Verification items for the finished model (mm, model axes). Give positions to 0.01 mm unless a question says otherwise; leave off trailing zeros. Loops run counter-clockwise (first coordinate to the right, second up) from the corner with the lowest first, then second, coordinate; pieces in that order, holes last. Notation, with made-up numbers: (72, 60.25) - (119, 60.25) arc R12 ccw to (119, 83.25) - close; hole circle Ø2 at (52.5, 35.5). An arc over 180 degrees is marked (long way). One line per question, with ' | ' between items. Start each with the question number.
1. Thickness scan on line 1 along Y through (x, z) = (0.55, -7) (3 decimals); line 2 along Z through (x, y) = (-0.5, -53.5); line 3 along Y through (x, z) = (0.6, -20) (3 decimals). Record the ranges inside material, lowest first. Write a range as from..to.
2. Depth check by flat-ended pin: pin 1 Ø2.5 at (y, z) = (-14.795, -13) entering from -X. Enter the tip coordinate at first touch or a pass-through.
3. Section check A-A, the plane z = -13. Enter the section's corners in (x, y) (3 decimals).
4. Section check D-D, the plane x = 0.05. Enter the section's corners in (y, z) (3 decimals).
5. Section check B-B, the plane z = -4. Enter the section's corners in (x, y) (3 decimals).
6. Section check C-C, the plane y = -54. Enter the section's corners in (x, z), then the cut area to 3 significant figures.
from build123d import *

# Parameters (mm, degrees)
EXTRUDE_1_DEPTH     = 2
FILLET_1_R          = 2
FILLET_2_R          = 2
FILLET_3_R          = 2
FILLET_4_R          = 2
SKETCH_2_W          = 12
SKETCH_2_H          = 89.95
EXTRUDE_2_DEPTH     = 2
CUT_EXTRUDE_1_DEPTH = 10
SKETCH_6_R          = 1.6
CUT_EXTRUDE_2_DEPTH = 10
SKETCH_7_W          = 10
SKETCH_7_H          = 89.95
EXTRUDE_3_DEPTH     = 2


with BuildPart() as part:
    # 草图1 → 凸台-拉伸1 (new body)
    with BuildSketch(Plane(origin=(-0.79375, 0, 0), x_dir=(0, -1, 0), z_dir=(-1, 0, 0))):
        with BuildLine():
            Line((38.795, 5), (12.795, 5))
            ThreePointArc((12.795, 5), (11.380786438, 4.414213562), (10.795, 3))
            Line((10.795, 3), (10.795, -13))
            ThreePointArc((10.795, -13), (11.380786438, -14.414213562), (12.795, -15))
            Line((12.795, -15), (47.795, -15))
            Line((47.795, -15), (50.77, -0.039144756))
            Line((50.77, -0.039144756), (55.77, -0.039144756))
            Line((55.77, -0.039144756), (60.77, -0.039144756))
            Line((60.77, -0.039144756), (63.745, -15))
            Line((63.745, -15), (98.745, -15))
            ThreePointArc((98.745, -15), (100.159213562, -14.414213562), (100.745, -13))
            Line((100.745, -13), (100.745, 3))
            ThreePointArc((100.745, 3), (100.159213562, 4.414213562), (98.745, 5))
            Line((98.745, 5), (72.745, 5))
            Line((72.745, 5), (38.795, 5))
        make_face()
    extrude(amount=-EXTRUDE_1_DEPTH)

    # 圆角1
    fillet_1_edges = [part.edges().sort_by_distance(p)[0] for p in [
        (0.20625, -47.795, -15),
    ]]
    fillet(fillet_1_edges, radius=FILLET_1_R)

    # 圆角2
    fillet_2_edges = [part.edges().sort_by_distance(p)[0] for p in [
        (0.20625, -50.77, -0.039144756),
    ]]
    fillet(fillet_2_edges, radius=FILLET_2_R)

    # 圆角3
    fillet_3_edges = [part.edges().sort_by_distance(p)[0] for p in [
        (0.20625, -60.77, -0.039144756),
    ]]
    fillet(fillet_3_edges, radius=FILLET_3_R)

    # 圆角4
    fillet_4_edges = [part.edges().sort_by_distance(p)[0] for p in [
        (0.20625, -63.745, -15),
    ]]
    fillet(fillet_4_edges, radius=FILLET_4_R)

    # 草图2 → 凸台-拉伸2 (add)
    with BuildSketch(Plane(origin=(1.20625, 0, 0), x_dir=(0, 0, -1), z_dir=(1, 0, 0))):
        with Locations((-9, -55.77)):
            Rectangle(SKETCH_2_W, SKETCH_2_H)
        Polygon((13.39006724, -48.115138781), (25, -45.806477318), (25, -10.795), (13, -10.795), align=None)
        Polygon((13.39006724, -63.424861219), (25, -65.733522682), (25, -100.745), (13, -100.745), align=None)
    extrude(amount=-EXTRUDE_2_DEPTH)

    # 草图5 → 切除-拉伸1 (cut)
    with BuildSketch(Plane(origin=(1.20625, 0, 0), x_dir=(0, 0, -1), z_dir=(1, 0, 0))):
        Polygon((1.649077515, -50.449861219), (25, -45.806477318), (25, -39.241825321), align=None)
        Polygon((1.649077515, -61.090138781), (25, -72.298174679), (25, -65.733522682), align=None)
    extrude(amount=-CUT_EXTRUDE_1_DEPTH, mode=Mode.SUBTRACT)

    # 草图6 → 切除-拉伸2 (cut)
    with BuildSketch(Plane(origin=(1.20625, 0, 0), x_dir=(0, 0, -1), z_dir=(1, 0, 0))):
        with Locations((13, -14.795)):
            Circle(SKETCH_6_R)
        with Locations((7, -14.795)):
            Circle(SKETCH_6_R)
        with Locations((13, -96.745)):
            Circle(SKETCH_6_R)
        with Locations((7, -96.745)):
            Circle(SKETCH_6_R)
    extrude(amount=-CUT_EXTRUDE_2_DEPTH, mode=Mode.SUBTRACT)

    # 草图7 → 凸台-拉伸3 (add)
    with BuildSketch(Plane.ZY.offset(0.79375)):
        with Locations((20, -55.77)):
            Rectangle(SKETCH_7_W, SKETCH_7_H)
    extrude(amount=-EXTRUDE_3_DEPTH)


solid = part.part
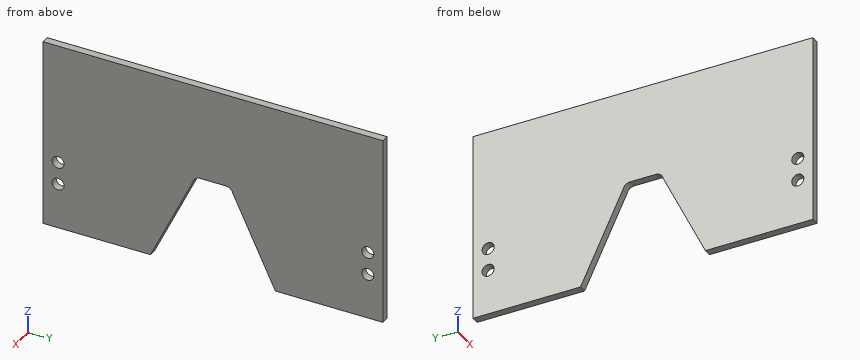
Results list:
1) line 1: -100.745..-98.345, -95.145..-63.658, -47.882..-16.395, -13.195..-10.795 | line 2: -0.04..25 | line 3: -100.745..-69.898, -41.642..-10.795
2) pin 1: through
3) outline: (-0.794, -100.745) - (1.206, -100.745) - (1.206, -98.345) - (-0.794, -98.345) - close; (-0.794, -95.145) - (1.206, -95.145) - (1.206, -66.538) - (-0.794, -66.538) - close; (-0.794, -45.002) - (1.206, -45.002) - (1.206, -16.395) - (-0.794, -16.395) - close; (-0.794, -13.195) - (1.206, -13.195) - (1.206, -10.795) - (-0.794, -10.795) - close
4) outline: (-100.745, -25) - (-72.298, -25) - (-61.09, -1.649) arc R2 cw to (-59.129, -0.039) - (-52.411, -0.039) arc R2 cw to (-50.45, -1.649) - (-39.242, -25) - (-10.795, -25) - (-10.795, 25) - (-100.745, 25) - close; hole circle Ø3.2 at (-96.745, -13); hole circle Ø3.2 at (-96.745, -7); hole circle Ø3.2 at (-14.795, -13); hole circle Ø3.2 at (-14.795, -7)
5) outline: (-0.794, -100.745) - (1.206, -100.745) - (1.206, -62.219) - (-0.794, -62.219) - close; (-0.794, -49.321) - (1.206, -49.321) - (1.206, -10.795) - (-0.794, -10.795) - close
6) outline: (-0.79, -0.04) - (1.21, -0.04) - (1.21, 25) - (-0.79, 25) - close | area: 50.1 mm²
